```python
from build123d import *

# Parameters (mm, degrees)
SKETCH2_R           = 5
BOSS_EXTRUDE1_DEPTH = 94.5
BOSS_EXTRUDE2_DEPTH = 30
CUT_EXTRUDE5_REACH  = 101.36
CUT_EXTRUDE1_DEPTH  = 30
SKETCH7_R           = 2.0000000000000027
CUT_EXTRUDE2_DEPTH  = 10
CIRPATTERN1_COUNT   = 3
CUT_EXTRUDE6_REACH  = 104.514
CUT_EXTRUDE7_REACH  = 105.272


with BuildPart() as part:
    # Sketch2 → Boss-Extrude1 (new body)
    with BuildSketch(Plane(origin=(0, 0, 0), x_dir=(1, 0, 0), z_dir=(0, 1, 0))):
        with Locations(Location((0, 0, 0), (0, 0, 270))):
            Circle(SKETCH2_R)
    extrude(amount=BOSS_EXTRUDE1_DEPTH)

    # Sketch3 → Boss-Extrude2 (add)
    with BuildSketch(Plane.XY):
        with BuildLine():
            Line((1.4999999999999998, 85), (1.500000000000006, 35))
            ThreePointArc((1.500000000000006, 35), (5.48e-15, 33.5), (-1.4999999999999942, 35))
            Line((-1.4999999999999942, 35), (-1.5000000000000007, 85))
            ThreePointArc((-1.5000000000000007, 85), (-2.8e-16, 86.5), (1.4999999999999998, 85))
        make_face()
    boss_extrude2 = extrude(amount=BOSS_EXTRUDE2_DEPTH)

    # Sketch12 → Cut-Extrude5 (cut, up to next)
    with BuildSketch(Plane.ZY.offset(1.4999999999999896), mode=Mode.PRIVATE) as cut_extrude5_sk1:
        Polygon((30, 86.50000000000001), (30, 76.50000000000001), (19, 86.50000000000001), align=None)
    cut_extrude5_tool1 = extrude(cut_extrude5_sk1.sketch, amount=-CUT_EXTRUDE5_REACH, mode=Mode.PRIVATE) & part.part
    # Sketch12 → Cut-Extrude5 (cut, up to next)
    with BuildSketch(Plane.ZY.offset(1.4999999999999896), mode=Mode.PRIVATE) as cut_extrude5_sk2:
        Polygon((30, 33.5), (19, 33.5), (30, 43.50000000000001), align=None)
    cut_extrude5_tool2 = extrude(cut_extrude5_sk2.sketch, amount=-CUT_EXTRUDE5_REACH, mode=Mode.PRIVATE) & part.part
    add(cut_extrude5_tool1.solids().sort_by_distance((-1.5, 83.166667, 26.333333))[0], mode=Mode.SUBTRACT)
    add(cut_extrude5_tool2.solids().sort_by_distance((-1.5, 36.833333, 26.333333))[0], mode=Mode.SUBTRACT)

    # Sketch6 → Cut-Extrude1 (cut)
    with BuildSketch(Plane(origin=(0, 94.5, 0), x_dir=(1, 0, 0), z_dir=(0, 1, 0))):
        with BuildLine():
            Line((0, 1.5), (1.4900443781608952, -0.1725333333333336))
            ThreePointArc((1.4900443781608952, -0.1725333333333336), (-1.1200000000000003, -0.9977975746613132), (0, 1.5))
        make_face()
    extrude(amount=-CUT_EXTRUDE1_DEPTH, mode=Mode.SUBTRACT)

    # Sketch7 → Cut-Extrude2 (cut)
    with BuildSketch(Plane.XY):
        with Locations(Location((0, 88.85909657897355, 0), (0, 0, 90))):
            Circle(SKETCH7_R)
    extrude(amount=-CUT_EXTRUDE2_DEPTH, mode=Mode.SUBTRACT)

    # CirPattern1: Boss-Extrude2 ×3 about axis
    cirpattern1_axis = Axis((-1e-16, 0, -4.9e-16), (0, 1, 0))
    for i in range(1, CIRPATTERN1_COUNT):
        add(boss_extrude2.rotate(cirpattern1_axis, i * 360 / CIRPATTERN1_COUNT))

    # Sketch13 → Cut-Extrude6 (cut, up to next)
    with BuildSketch(Plane(origin=(0.7499999999999831, -2e-16, 1.2990381056766571), x_dir=(0.8660254037844431, 0, -0.499999999999992), z_dir=(0.49999999999999206, 0, 0.8660254037844433)), mode=Mode.PRIVATE) as cut_extrude6_sk1:
        Polygon((30.00000000000001, 86.50000000000001), (30.000000000000014, 76.50000000000001), (19.00000000000001, 86.50000000000001), align=None)
    cut_extrude6_tool1 = extrude(cut_extrude6_sk1.sketch, amount=-CUT_EXTRUDE6_REACH, mode=Mode.PRIVATE) & part.part
    # Sketch13 → Cut-Extrude6 (cut, up to next)
    with BuildSketch(Plane(origin=(0.7499999999999831, -2e-16, 1.2990381056766571), x_dir=(0.8660254037844431, 0, -0.499999999999992), z_dir=(0.49999999999999206, 0, 0.8660254037844433)), mode=Mode.PRIVATE) as cut_extrude6_sk2:
        Polygon((30.00000000000001, 33.5), (19.00000000000001, 33.50000000000001), (30.000000000000007, 43.50000000000001), align=None)
    cut_extrude6_tool2 = extrude(cut_extrude6_sk2.sketch, amount=-CUT_EXTRUDE6_REACH, mode=Mode.PRIVATE) & part.part
    add(cut_extrude6_tool1.solids().sort_by_distance((23.555336, 83.166667, -11.867629))[0], mode=Mode.SUBTRACT)
    add(cut_extrude6_tool2.solids().sort_by_distance((23.555336, 36.833333, -11.867629))[0], mode=Mode.SUBTRACT)

    # Sketch14 → Cut-Extrude7 (cut, up to next)
    with BuildSketch(Plane(origin=(0.7500000000000019, -2e-16, -1.2990381056766473), x_dir=(-0.8660254037844363, 0, -0.5000000000000043), z_dir=(0.5000000000000042, 0, -0.8660254037844362)), mode=Mode.PRIVATE) as cut_extrude7_sk1:
        Polygon((29.999999999999986, 86.50000000000001), (29.99999999999993, 76.50000000000001), (18.999999999999986, 86.50000000000001), align=None)
    cut_extrude7_tool1 = extrude(cut_extrude7_sk1.sketch, amount=-CUT_EXTRUDE7_REACH, mode=Mode.PRIVATE) & part.part
    # Sketch14 → Cut-Extrude7 (cut, up to next)
    with BuildSketch(Plane(origin=(0.7500000000000019, -2e-16, -1.2990381056766473), x_dir=(-0.8660254037844363, 0, -0.5000000000000043), z_dir=(0.5000000000000042, 0, -0.8660254037844362)), mode=Mode.PRIVATE) as cut_extrude7_sk2:
        Polygon((29.999999999999993, 33.5), (18.999999999999993, 33.50000000000001), (29.999999999999986, 43.50000000000001), align=None)
    cut_extrude7_tool2 = extrude(cut_extrude7_sk2.sketch, amount=-CUT_EXTRUDE7_REACH, mode=Mode.PRIVATE) & part.part
    add(cut_extrude7_tool1.solids().sort_by_distance((-22.055336, 83.166667, -14.465705))[0], mode=Mode.SUBTRACT)
    add(cut_extrude7_tool2.solids().sort_by_distance((-22.055336, 36.833333, -14.465705))[0], mode=Mode.SUBTRACT)


solid = part.part
```
Check sheet for the modelled part. Datum: model origin and axes. Units: mm. A direction names the side the tool comes from. Round coordinates to 2 decimals unless told otherwise and drop trailing zeros. Write each loop counter-clockwise with the first axis right and the second up, starting at its lowest first coordinate (ties: lowest second). Pieces come first, ordered by that corner, then holes. Notation, with made-up numbers: (37, 67.5) -> (74, 67.5) arc R21 ccw to (74, 83.5) -> close; hole circle Ø11 at (76, 29). An arc over 180 degrees is marked (long way). Put each result on its own line as item: value.
(1) Sectioned sample at C-C (z = 14). Enter the section's corners in (x, y), plus the area to 3 significant figures.
Values found:
outline: (-1.5, 35) arc R1.5 ccw to (1.5, 35) -> (1.5, 85) arc R1.5 ccw to (-1.5, 85) -> close
area: 157 mm^2
(2) Sectioned sample at A-A (y = 75). Enter the section's corners in (x, z), plus the area to 3 significant figures.
Values found:
outline: (-26.73, -13.7) -> (-25.23, -16.3) -> (-3.38, -3.68) arc R5 ccw to (3.38, -3.68) -> (25.23, -16.3) -> (26.73, -13.7) -> (4.88, -1.09) arc R5 ccw to (1.5, 4.77) -> (1.5, 30) -> (-1.5, 30) -> (-1.5, 4.77) arc R5 ccw to (-4.88, -1.09) -> close; hole (-0.75, 1.3) -> (0, 0) -> (0.75, 1.3) arc R1.5 ccw to start
area: 303 mm^2
(3) Tool access check on faces 5 (the face through (0, 33.5, 12.6)), 6 (the face through (1.5, 60, 17)), 7 (the face through (14.15, 60.35, -9.9)), 8 (the face through (-1.5, 60, 17)), 9 (the face through (0, 86.5, 12.6)). Record the directions out of +Z, -Z, +X, -X, +Y, -Y that give a thin tool (end or side, any length) a straight path to the whole face; none if there is none.
Values found:
face 5: +Z, -Y
face 6: +Z, +X, +Y, -Y
face 7: -Z, +Y, -Y
face 8: +Z, -X, +Y, -Y
face 9: +Z, +Y
(4) Mould release check, pull along Y, two halves, no side actions. Record for faces 1 (the face through (-10.9, 86.5, -6.3)), 2 (the face through (-21.14, 38.43, -12.23)), 3 (the face through (-25.99, 60.23, -14.98)), 4 (the face through (1.952, 88.426, -2.467)): released by +Y, released by -Y, zero draft, split by the parting line, or undercut.
Values found:
face 1: released by +Y
face 2: released by -Y
face 3: zero draft
face 4: undercut
(5) Material ranges on line 1 (X direction, y = 8.5, z = 0); line 2 (X direction, y = 85, z = 12); line 3 (Z direction, x = 1, y = 13), recorded low to high.
Values found:
line 1: x = -5 to 5
line 2: x = -1.5 to 1.5
line 3: z = -4.9 to 4.9
(6) Go/stop test with flat-tipped pins: pin 1 Ø4 at (x, y) = (-19.5, 74.5) entering from -Z; pin 2 Ø10 at (x, z) = (4, -4.5) entering from +Y; pin 3 Ø12 at (x, y) = (-15, 77.5) entering from -Z; pin 4 Ø3 at (x, y) = (-4.5, 84) entering from +Z. Record where each tip stops, or that it passes through.
Values found:
pin 1: stops at z = -14.15
pin 2: stops at y = 94.5
pin 3: stops at z = -13.86
pin 4: stops at z = 4
(7) Sectioned sample at D-D (y = 38.5). Enter the section's corners in (x, z).
Values found:
outline: (-21.97, -10.95) -> (-20.47, -13.55) -> (-3.38, -3.68) arc R5 ccw to (3.38, -3.68) -> (20.47, -13.55) -> (21.97, -10.95) -> (4.88, -1.09) arc R5 ccw to (1.5, 4.77) -> (1.5, 24.5) -> (-1.5, 24.5) -> (-1.5, 4.77) arc R5 ccw to (-4.88, -1.09) -> close
(8) Sectioned sample at B-B (y = 54). Enter the section's corners in (x, z), plus the area to 3 significant figures.
Values found:
outline: (-26.73, -13.7) -> (-25.23, -16.3) -> (-3.38, -3.68) arc R5 ccw to (3.38, -3.68) -> (25.23, -16.3) -> (26.73, -13.7) -> (4.88, -1.09) arc R5 ccw to (1.5, 4.77) -> (1.5, 30) -> (-1.5, 30) -> (-1.5, 4.77) arc R5 ccw to (-4.88, -1.09) -> close
area: 304 mm^2
